Input: part model. Units: mm. Frame: model coordinates. Face numbers are marked on the shaded views. Coordinates: 2 decimals unless noted, no trailing zeros. Loops run counter-clockwise (first coordinate to the right, second up) from the corner with the lowest first, then second, coordinate; pieces in that order, holes last.
(1) Mould query, pull axis Z, two halves, no side actions, for the marked faces 1 and 2. Classes: released by +Z, released by -Z, zero draft, split by the parting line, or undercut.
(2) Section D-D, the plane z = 0. Return loops of the section in (x, y).
(3) Contact query for flat-ended pins moving along their axis: P1, Ø8, axis at y = 3, z = -15.5, coming from the -X side; P2, Ø3, axis at x = 5, z = 10, coming from the +Y side; P3, Ø8, axis at y = 8, z = 10, coming from the +X side. Output: stop coordinate, or through.
(4) Line query: L1, parallel to X at y = 3.7, z = 0; L2, parallel to Z at x = -1.5, y = 13.5; L3, parallel to Y at x = 2.5, z = 8.5. Output: solid intervals per line, ascending.
(5) Section B-B, the plane z = 20. Return loops of the section in (x, y), then the cut area to 3 significant figures.
(6) Section A-A, the plane x = -20. Return loops of the section in (y, z).
(7) Section C-C, the plane x = 0. Return loops of the section in (y, z), then the cut area to 3 significant figures.
```python
from build123d import *

# Parameters (mm, degrees)
SKETCH1_R           = 25
SKETCH1_R_2         = 1.5
BOSS_EXTRUDE1_DEPTH = 5
SKETCH2_R           = 2.5
BOSS_EXTRUDE2_DEPTH = 14
SKETCH3_R           = 1.5
CUT_EXTRUDE1_DEPTH  = 5
CUT_EXTRUDE3_START  = -13.9
CUT_EXTRUDE3_DEPTH  = 13.9


with BuildPart() as part:
    # Sketch1 → Boss-Extrude1 (new body)
    with BuildSketch(Plane(origin=(0, 0, 0), x_dir=(1, 0, 0), z_dir=(0, 1, 0))):
        with Locations(Location((0, 0, 0), (0, 0, 270))):
            Circle(SKETCH1_R)
        with Locations(Location((0, -20, 0), (0, 0, 270))):
            Circle(SKETCH1_R_2, mode=Mode.SUBTRACT)
        with Locations(Location((-20, 0, 0), (0, 0, 270))):
            Circle(SKETCH1_R_2, mode=Mode.SUBTRACT)
        with Locations(Location((0, 20, 0), (0, 0, 270))):
            Circle(SKETCH1_R_2, mode=Mode.SUBTRACT)
        with Locations(Location((20, 0, 0), (0, 0, 270))):
            Circle(SKETCH1_R_2, mode=Mode.SUBTRACT)
    extrude(amount=BOSS_EXTRUDE1_DEPTH)

    # Sketch2 → Boss-Extrude2 (add)
    with BuildSketch(Plane(origin=(0, 5, 0), x_dir=(1, 0, 0), z_dir=(0, 1, 0))):
        with Locations(Location((0, 0, 0), (0, 0, 270))):
            Circle(SKETCH2_R)
    extrude(amount=BOSS_EXTRUDE2_DEPTH)

    # Sketch3 → Cut-Extrude1 (cut)
    with BuildSketch(Plane.XZ):
        with Locations(Location((0, 0, 0), (0, 0, 270))):
            Circle(SKETCH3_R)
    extrude(amount=-CUT_EXTRUDE1_DEPTH, mode=Mode.SUBTRACT)

    # Sketch4 → Cut-Extrude3 (cut)
    with BuildSketch(Plane(origin=(0, 19, 0), x_dir=(1, 0, 0), z_dir=(0, 1, 0)).offset(CUT_EXTRUDE3_START)):
        with BuildLine():
            Line((2, -1.5), (-2, -1.5))
            ThreePointArc((-2, -1.5), (0, -2.5), (2, -1.5))
        make_face()
    extrude(amount=CUT_EXTRUDE3_DEPTH, mode=Mode.SUBTRACT)


solid = part.part
```
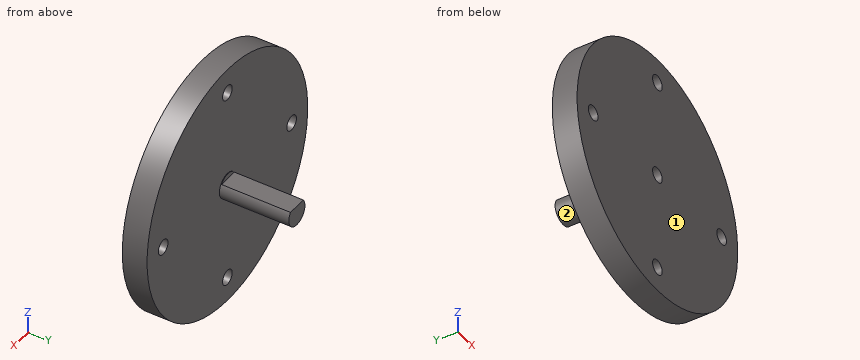
Report:
1. face 1: zero draft
1. face 2: split by the parting line
2. outline: (-25, 0) - (-21.5, 0) - (-21.5, 5) - (-25, 5) - close; (-18.5, 0) - (-1.5, 0) - (-1.5, 5) - (1.5, 5) - (1.5, 0) - (18.5, 0) - (18.5, 5) - (2.5, 5) - (2.5, 19) - (-2.5, 19) - (-2.5, 5) - (-18.5, 5) - close; (21.5, 0) - (25, 0) - (25, 5) - (21.5, 5) - close
3. P1: stops at x = -22.2
3. P2: stops at y = 5
3. P3: stops at x = 23.89
4. L1: x = -25 to -21.5, -18.5 to -1.5, 1.5 to 18.5, 21.5 to 25
4. L2: z = -2 to 1.5
4. L3: y = 0 to 5
5. outline: (-15, 0) - (-1.5, 0) - (-1.5, 5) - (-15, 5) - close; (1.5, 0) - (15, 0) - (15, 5) - (1.5, 5) - close
5. area: 135 mm2
6. outline: (0, -15) - (5, -15) - (5, -1.5) - (0, -1.5) - close; (0, 1.5) - (5, 1.5) - (5, 15) - (0, 15) - close
7. outline: (0, -25) - (5, -25) - (5, -21.5) - (0, -21.5) - close; (0, -18.5) - (5, -18.5) - (5, -2.5) - (19, -2.5) - (19, 1.5) - (5.1, 1.5) - (5.1, 2.5) - (5, 2.5) - (5, 18.5) - (0, 18.5) - (0, 1.5) - (5, 1.5) - (5, -1.5) - (0, -1.5) - close; (0, 21.5) - (5, 21.5) - (5, 25) - (0, 25) - close
7. area: 261 mm2
